Geometry: see drawing. Coordinates: mm, zero at the bounding-box minimum. A direction names the side the tool comes from. Round coordinates to 2 decimals unless told otherwise and drop trailing zeros. Loops run counter-clockwise (first coordinate to the right, second up) from the corner with the lowest first, then second, coordinate; pieces in that order, holes last.
(1) Mould query, pull axis Y, two halves, no side actions, for the marked faces 4, 5, 6 and 7. Classes: pulls with the +Y half, pulls with the -Y half, needs draft (parallel to the pull), parting line crosses it, or undercut.
(2) Section D-D, the plane x = 7.5. Return the cut outline in (y, z), plus the area to 3 significant figures.
(3) Set-up query: the marked faces 1, 2 and 3. Return all of +Z, -Z, +X, -X, +Y, -Y with unobstructed straight access to the full face (end or side cutting, diameter ignored); none if empty.
(4) Section A-A, the plane x = 5. Return the cut outline in (y, z).
(5) Material intervals for probe 1 along Y at (x, z) = (3.25, 16.25); probe 2 along X at (y, z) = (4, 5.75); probe 3 along X at (y, z) = (7.25, 4), sorted ascending.
(6) Section B-B, the plane y = 5.75. Return the cut outline in (x, z).
(7) Section C-C, the plane z = 14.5. Return the cut outline in (x, y).
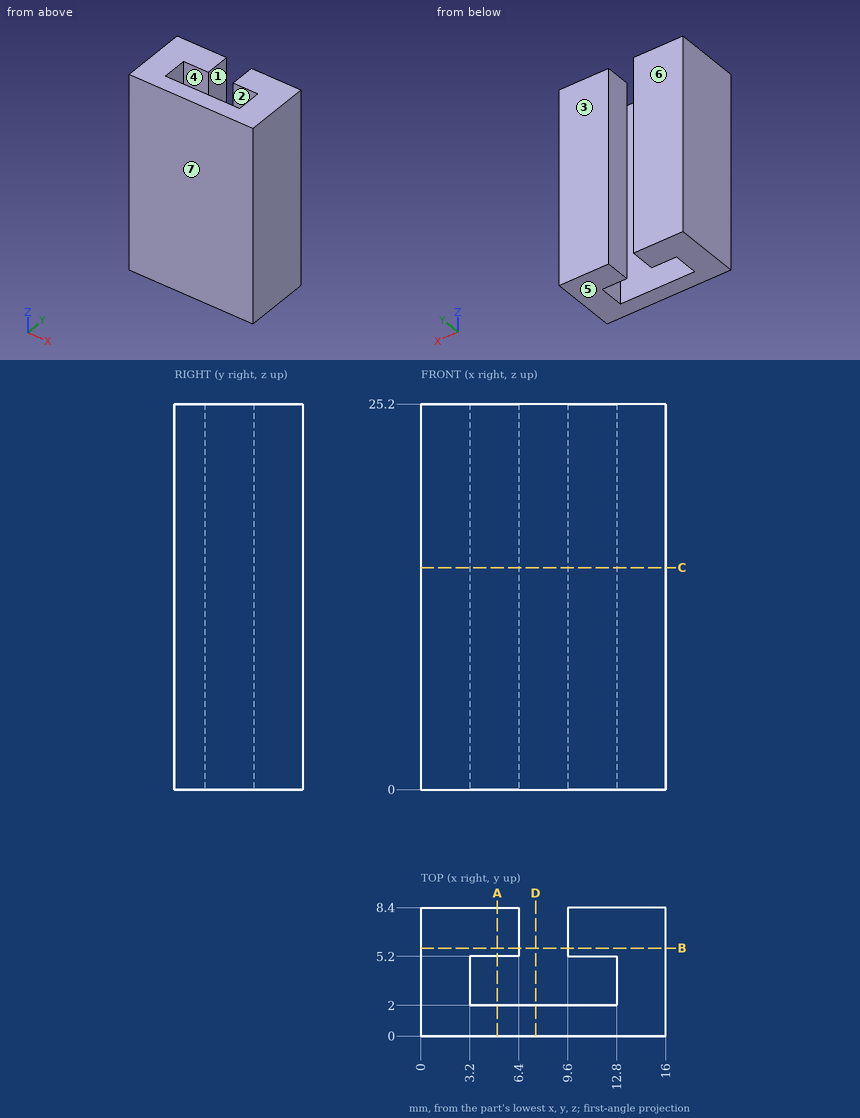
Output values:
1. face 4: undercut
1. face 5: needs draft
1. face 6: pulls with the +Y half
1. face 7: pulls with the -Y half
2. outline: (0, 0) - (2, 0) - (2, 25.2) - (0, 25.2) - close
2. area: 50.4 mm2
3. face 1: +Z, -Z, +Y
3. face 2: +Z, -Z
3. face 3: +Z, -Z, +X, -X, +Y
4. outline: (0, 0) - (2, 0) - (2, 25.2) - (0, 25.2) - close; (5.2, 0) - (8.4, 0) - (8.4, 25.2) - (5.2, 25.2) - close
5. probe 1: y = 0 to 2, 5.2 to 8.4
5. probe 2: x = 0 to 3.2, 12.8 to 16
5. probe 3: x = 0 to 6.4, 9.6 to 16
6. outline: (0, 0) - (6.4, 0) - (6.4, 25.2) - (0, 25.2) - close; (9.6, 0) - (16, 0) - (16, 25.2) - (9.6, 25.2) - close
7. outline: (0, 0) - (16, 0) - (16, 8.4) - (9.6, 8.4) - (9.6, 5.2) - (12.8, 5.2) - (12.8, 2) - (3.2, 2) - (3.2, 5.2) - (6.4, 5.2) - (6.4, 8.4) - (0, 8.4) - close
